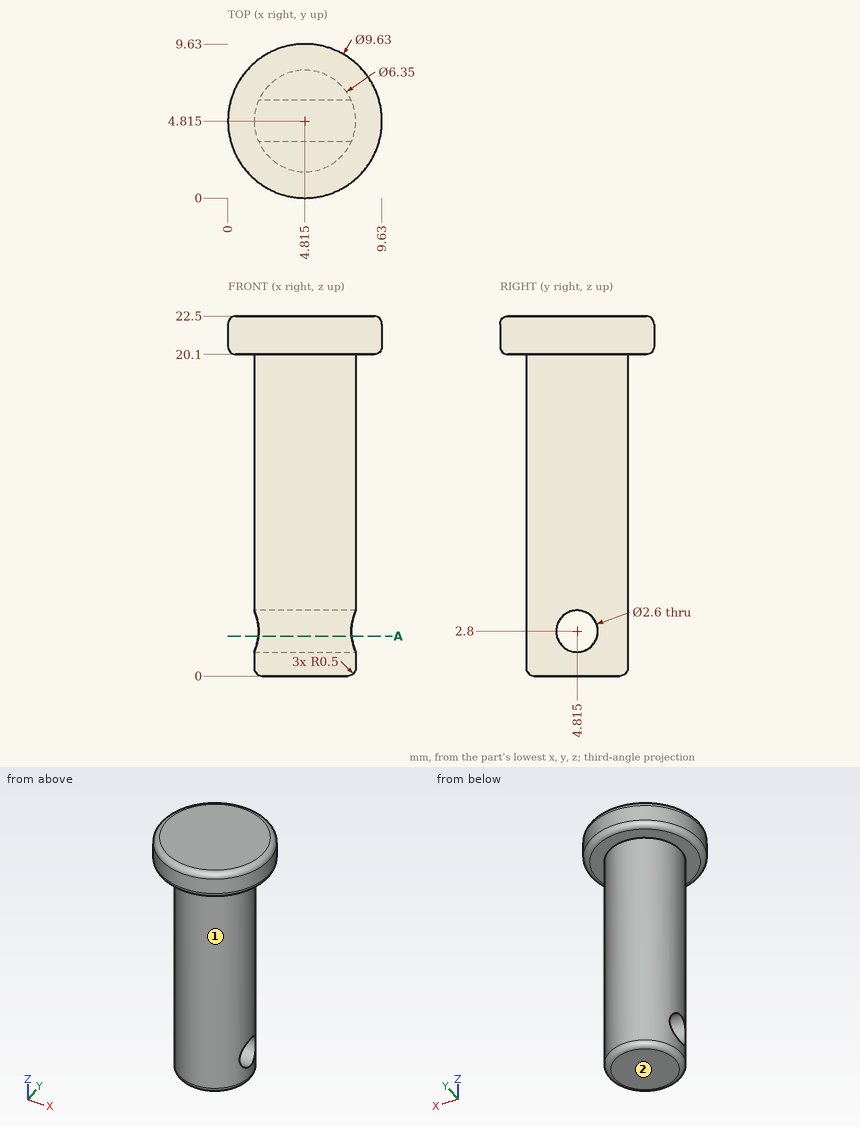
Drawing for the job (mm, zero at the part's lowest x, y, z). A direction names the side the tool comes from. Coordinates: 2 decimals unless noted, no trailing zeros. Order: outer loops, then holes, each group sorted by start corner. A loop starts at its lowest first (then second) coordinate and runs counter-clockwise, first axis right, second up. Notation, with made-up numbers: (-3, 7) -> (42, 7) arc R9 ccw to (42, 16) -> close; hole circle Ø6 at (64, -31.75). An arc over 180 degrees is marked (long way). One line per item, written item: value.
(1) Drop flat-ended pins along their axis: pin 1 Ø1 at (y, z) = (8, 13.5) entering from +X; pin 2 Ø4 at (y, z) = (6, 6) entering from +X; pin 3 Ø2.5 at (y, z) = (4.815, 2.8) entering from -X; pin 4 Ø1.5 at (x, z) = (8, 16) entering from -Y. Give the stop position or say it passes through.
Checked values:
pin 1: x = 6.51
pin 2: x = 7.99
pin 3: through
pin 4: y = 2.78
(2) Slice it at A-A, the plane z = 2.5. List the corners of the cut face in (x, y) (3 decimals), plus the area to 3 significant figures.
Checked values:
outline: (1.903, 3.55) arc R3.175 ccw to (7.727, 3.55) -> close; (1.903, 6.08) -> (7.727, 6.08) arc R3.175 ccw to start
area: 16.0 mm2
(3) Tool access for the marked faces 1 and 2: list every direction of +Z, -Z, +X, -X, +Y, -Y with a clear straight run to the whole face (end or side of a thin tool).
Checked values:
face 1: -Z
face 2: -Z, +X, -X, +Y, -Y
(4) Probe line 1 (Z direction, x = 5.75, y = 4.75); line 2 (Z direction, x = 7.25, y = 2.5); line 3 (Y direction, x = 4.5, z = 2.8) (3 decimals). List the from-to ranges inside material, lowest first. Write a range as [from, to].
Checked values:
line 1: [0, 1.5], [4.1, 22.5]
line 2: [20.1, 22.5]
line 3: [1.656, 3.515], [6.115, 7.974]
